Can you work these out from the model? Positions are in its coordinate system, mm. A direction names the side the tool comes from. Give positions to 0.01 mm unless a question says otherwise; leave off trailing zeros. Order: outer loops, then holes, each group sorted by start corner. A loop starts at its lowest first (then second) coordinate and runs counter-clockwise, first axis right, second up. Notation, with made-up numbers: (37, -28.75) -> (91, -28.75) arc R11 cw to (91, -10.75) -> close; hole circle Ø3 at (38, 63). An arc over 180 degrees is marked (long way). Answer as CSV lines item,"result".
Autodesk Fusion 360 part; units mm, degrees
sketch "Sketch1" plane through (0, 0, 0) normal (0, 1, 0) x (1, 0, 0)
  circle A0 centre (0, 0) radius 5
  dimension "d1" = 10
extrude "Extrude1" add sketch "Sketch1" along normal blind 5
sketch "Sketch2" plane through (0, 5, 0) normal (0, 1, 0) x (-1, 0, 0)
  circle A0 centre (0, 0) radius 5
  line L0 (-1.25, -5) -> (1.25, -5)
  line L1 (1.25, -5) -> (1.25, 5)
  line L2 (1.25, 5) -> (-1.25, 5)
  line L3 (-1.25, 5) -> (-1.25, -5)
  line L4 (-1.25, -5) -> (1.25, 5) construction
  line L5 (1.25, -5) -> (-1.25, 5) construction
  dimension "d4" = 2.5
  dimension "d5" = 10
extrude "Extrude2" add sketch "Sketch2" along normal blind 3 contours A0 L1 L3
sketch "Sketch3" plane through (0, 0, 0) normal (0, -1, 0) x (1, 0, 0)
  circle A0 centre (0, 0) radius 5
  circle A1 centre (0, 0) radius 5.75
  dimension "d8" = 11.5
extrude "Extrude3" add sketch "Sketch3" along normal blind 2 contours A0 | A1
sketch "Sketch5" plane through (0, -2, 0) normal (0, -1, 0) x (1, 0, 0)
  circle A0 centre (0, 0) radius 5.75
  circle A1 centre (0, 0) radius 2
  dimension "d11" = 4
extrude "Extrude4" cut sketch "Sketch5" against normal blind 6.5 contours A1
Item 1: Imagine slicing it at C-C, the plane y = -1.5. Please give me the cut outline in (x, z).
Numbers:
outline,"circle Ø11.5 at (0, 0); hole circle Ø4 at (0, 0)"
Item 2: Imagine slicing it at D-D, the plane z = -2.5. Please give me the cut outline in (x, y), then the cut area to 3 significant figures.
Numbers:
outline,"(-5.18, -2) -> (5.18, -2) -> (5.18, 0) -> (4.33, 0) -> (4.33, 5) -> (1.25, 5) -> (1.25, 8) -> (-1.25, 8) -> (-1.25, 5) -> (-4.33, 5) -> (-4.33, 0) -> (-5.18, 0) -> close"
area,"71.5 mm²"
Item 3: For faces 1 (the flat face through (-1.25, 6, 0)), 2 (the cylindrical face through (-5, 3, 0)), 3 (the flat face through (3, 5, 0)), 4 (the flat face through (0, 8, 0)), 5 (the flat face through (2.5, -2, 0.1)), which set-ups out of +Z, -Z, +X, -X, +Y, -Y let a thin tool reach every point of the face, with its end or its side?
Numbers:
face 1,"+Z, -Z, -X, +Y"
face 2,"+Y"
face 3,"+Z, -Z, +X, +Y"
face 4,"+Z, -Z, +X, -X, +Y"
face 5,"+Z, -Z, +X, -X, -Y"
Item 4: We'd pull the mould along X, two halves only. Please class faces 6 (the cylindrical face through (0, 1, -2)), 7 (the flat face through (-2, 0, 5)), 8 (the cylindrical face through (-0.75, -0.99, -5.7)), 9 (the flat face through (0, 4.5, 0)): released by +X, released by -X, zero draft, split by the parting line, or undercut.
Numbers:
face 6,"undercut"
face 7,"zero draft"
face 8,"split by the parting line"
face 9,"undercut"
Item 5: For pin 1 (1.5 mm diameter, centred on y = 7, z = -2, fed in from +X); pin 2 (2 mm diameter, centred on x = -3.5, z = 0, fed in from +Y); pin 3 (2 mm diameter, centred on x = 1.5, y = 0.5, fed in from +Z); pin 4 (4 mm diameter, centred on x = -2.5, z = 1, fed in from +Y), each with a flat end and sliding along its axis, tell me the tip position at first contact or that it passes through.
Numbers:
pin 1,"stops at x = 1.25"
pin 2,"stops at y = 5"
pin 3,"stops at z = 5.71"
pin 4,"stops at y = 8"
Item 6: Imagine slicing it at A-A, the plane x = 0. Please give me the cut outline in (y, z), then the cut area to 3 significant figures.
Numbers:
outline,"(-2, -5.75) -> (0, -5.75) -> (0, -5) -> (8, -5) -> (8, 5) -> (0, 5) -> (0, 5.75) -> (-2, 5.75) -> (-2, 2) -> (4.5, 2) -> (4.5, -2) -> (-2, -2) -> close"
area,"77.0 mm²"
Item 7: Imagine slicing it at B-B, the plane z = 0. Please give me the cut outline in (x, y).
Numbers:
outline,"(-5.75, -2) -> (-2, -2) -> (-2, 4.5) -> (2, 4.5) -> (2, -2) -> (5.75, -2) -> (5.75, 0) -> (5, 0) -> (5, 5) -> (1.25, 5) -> (1.25, 8) -> (-1.25, 8) -> (-1.25, 5) -> (-5, 5) -> (-5, 0) -> (-5.75, 0) -> close"
Item 8: Please list where these lines run through material, in increasing order: line 1 along Z through (x, y) = (0, 1.75); line 2 along Y through (x, z) = (-0.75, 5.25); line 3 along Y through (x, z) = (-2.5, -3.25).
Numbers:
line 1,"z = -5 to -2, 2 to 5"
line 2,"y = -2 to 0"
line 3,"y = -2 to 5"
